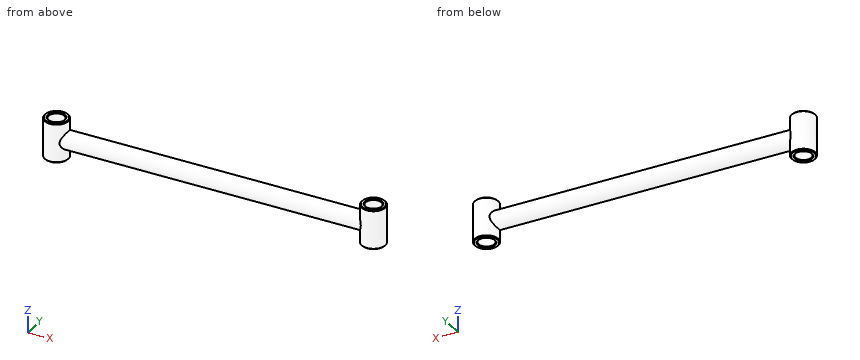
```python
from build123d import *

# Parameters (mm, degrees)
F0_R     = 19.05
F1_DEPTH = 63.5
F3_R     = 14.2875
F5_R     = 12.7
F6_DEPTH = 63.5
F7_SIZE  = 1.27


with BuildPart() as f1:
    # F0 (on Top) → F1 (new body)
    with BuildSketch(Plane.XY):
        Circle(F0_R)
        with Locations((508, 0)):
            Circle(F0_R)
    extrude(amount=F1_DEPTH)

    # F4: sweep along a path in F2
    with BuildLine(Plane.XZ) as f4_path:
        Line((0, 31.75), (508, 31.75))
    # F3 (on Right) → F4 (sweep)
    with BuildSketch(Plane.YZ):
        with Locations((0, 31.75)):
            Circle(F3_R)
    sweep(path=f4_path.line)

    # F5 (on face) → F6 (cut)
    with BuildSketch(Plane.XY.offset(63.5)):
        Circle(F5_R)
        with Locations((508, 0)):
            Circle(F5_R)
    extrude(amount=-F6_DEPTH, mode=Mode.SUBTRACT)

    # F7
    f7_edges = [f1.edges().sort_by_distance(p)[0] for p in [
        (-19.05, 0, 63.5),
        (-12.7, 0, 63.5),
        (-19.05, 0, 0),
        (-12.7, 0, 0),
        (488.95, 0, 0),
        (495.3, 0, 0),
        (495.3, 0, 63.5),
        (488.95, 0, 63.5),
    ]]
    chamfer(f7_edges, length=F7_SIZE)


solid = f1.part
```
The listing builds one solid part. Answer for the finished solid, in the listing's coordinates (mm). Coordinates: 2 decimals unless noted, no trailing zeros. Loops run counter-clockwise (first coordinate to the right, second up) from the corner with the lowest first, then second, coordinate; pieces in that order, holes last. Notation, with made-up numbers: (53.25, 36.5) -> (60.25, 36.5) arc R30 cw to (60.25, 60.5) -> close; hole circle Ø6 at (2, 30). An arc over 180 degrees is marked (long way). Use one line per item in the form item = value. Start each with the question number.
Item 1: The part is cut by section B-B on z = 56.5. Determine the outline of the cut face in (x, y), then the cut area to 3 significant figures.
Item 2: The part is cut by section A-A on x = 0. Determine the outline of the cut face in (y, z), then the cut area to 3 significant figures.
Item 3: Consider L1, parallel to Y at x = 508, z = 17; L2, parallel to X at y = 2, z = 48.5; L3, parallel to X at y = -7, z = 23. Determine where each line is inside the solid, lowest interval first. Write a range as [from, to].
Item 4: Flat-ended cylindrical pins translate along their axes: pin 1 Ø12 at (x, y) = (304.5, -12) entering from -Z; pin 2 Ø4 at (x, y) = (219.5, -6) entering from +Z; pin 3 Ø3 at (x, z) = (373, 35) entering from -Y. Find the tip coordinate at first contact, or state that the pin passes through.
Item 5: The part is cut by section C-C on z = 31.75. Determine the outline of the cut face in (x, y), then the cut area to 3 significant figures.
Answer key:
q1.outline = circle Ø38.1 at (0, 0); circle Ø38.1 at (508, 0); hole circle Ø25.4 at (0, 0); hole circle Ø25.4 at (508, 0)
q1.area = 1,270 mm2
q2.outline = (-19.05, 1.27) -> (-17.78, 0) -> (-13.97, 0) -> (-12.7, 1.27) -> (-12.7, 62.23) -> (-13.97, 63.5) -> (-17.78, 63.5) -> (-19.05, 62.23) -> close; (12.7, 1.27) -> (13.97, 0) -> (17.78, 0) -> (19.05, 1.27) -> (19.05, 62.23) -> (17.78, 63.5) -> (13.97, 63.5) -> (12.7, 62.23) -> close
q2.area = 800 mm2
q3.L1 = [-19.05, -12.7], [12.7, 19.05]
q3.L2 = [-18.94, -12.54], [12.54, 18.94], [489.06, 495.46], [520.54, 526.94]
q3.L3 = [-17.72, -10.6], [10.6, 497.4], [518.6, 525.72]
q4.pin_1 = 18.78
q4.pin_2 = 45.47
q4.pin_3 = -14.18
q5.outline = (12.6, -14.29) -> (495.4, -14.29) arc R19.05 ccw (long way) to (495.4, 14.29) -> (12.6, 14.29) arc R19.05 ccw (long way) to start; hole circle Ø25.4 at (0, 0); hole circle Ø25.4 at (508, 0)
q5.area = 14,800 mm2
